Verification items for the finished model (mm, model axes). Round coordinates to 2 decimals unless told otherwise and drop trailing zeros. Write each loop counter-clockwise with the first axis right and the second up, starting at its lowest first coordinate (ties: lowest second). Pieces come first, ordered by that corner, then holes. Notation, with made-up numbers: (-37.75, -39.75) - (19.25, -39.75) arc R20 cw to (19.25, -12.75) - close; hole circle Ø1 at (27, 40.25). An arc over 180 degrees is marked (long way). Answer as a JSON object with one key per item and string values.
Autodesk Inventor part; units mm, degrees
ref_plane "YZ Plane" through (0, 0, 0) normal (1, 0, 0) x (0, 1, 0)
ref_plane "XZ Plane" through (0, 0, 0) normal (0, 1, 0) x (-1, 0, 0)
ref_plane "XY Plane" through (0, 0, 0) normal (0, 0, 1) x (1, 0, 0)
sketch "Sketch1" plane through (0, 0, 0) normal (0, 0, 1) x (1, 0, 0)
  line L0 (700, -200) -> (180, -200)
  line L1 (180, -200) -> (-160, -200)
  line L2 (-160, -200) -> (-160, 200)
  line L3 (180, -200) -> (180, 200)
  line L4 (700, -200) -> (1018.8395, -200)
  line L5 (1018.8395, -200) -> (1018.8395, 200)
  line L6 (1018.8395, 200) -> (700, 200)
  line L7 (180, 200) -> (700, 200)
  line L8 (-160, 200) -> (180, 200)
  line L9 (740, 160) -> (740, 200)
  line L10 (740, 160) -> (740, -160)
  line L11 (740, -200) -> (740, -160)
  line L12 (700, 160) -> (700, -160)
  line L13 (700, -160) -> (700, -200)
  line L14 (700, 200) -> (700, 160)
  line L15 (140, 160) -> (140, 200)
  line L16 (140, -200) -> (140, -160)
  line L17 (140, 160) -> (140, -160)
  line L18 (700, -160) -> (180, -160)
  line L19 (180, 160) -> (700, 160)
  line L20 (180, -200) -> (340, -200)
  line L21 (340, -200) -> (340, 0)
  line L22 (340, 0) -> (180, 0)
  line L23 (180, 0) -> (180, -200)
  point P0 (0, 0)
  point P1 (260, 0)
  point P2 (140, 0)
  dimension "d0" = 160
extrude "Extrusion1" add sketch "Sketch1" along normal blind 160 contours L0 L3 L18 L21 | L18 L3 L22 L21
ref_plane "Work Plane1" through (260, -200, 0) normal (1, 0, 0) x (0, 0, -1)
sketch "Sketch2" plane through (260, -200, 0) normal (1, 0, 0) x (0, 0, -1)
  line L0 (0, 200) -> (0, 0)
  line L1 (0, 0) -> (-160, 0)
  line L2 (-160, 200) -> (-160, 0)
  line L3 (0, 200) -> (-160, 200)
  line L4 (0, 0) -> (-160, 0)
  line L5 (-80, 0) -> (-80, 200)
  line L6 (0, 200) -> (-160, 200)
  line L7 (-74, 200) -> (-74, 220)
  line L8 (-74, 220) -> (-50, 220)
  line L9 (-50, 220) -> (-50, 228)
  line L10 (-50, 228) -> (-80, 228)
  line L11 (-80, 228) -> (-80, 200)
  line L12 (-80, 200) -> (-80, 294.9893)
  dimension "d6" = 8
  dimension "d7" = 12
  dimension "d8" = 20
  dimension "d9" = 30
  dimension "d10" = 94.9893
revolve "Revolution1" add sketch "Sketch2" angle 360 about axis through (260, 0, 80) along (0, 1, 0) contours L3 L11 L10 L9 L8 L7
properties part number "aandrijfMotor"
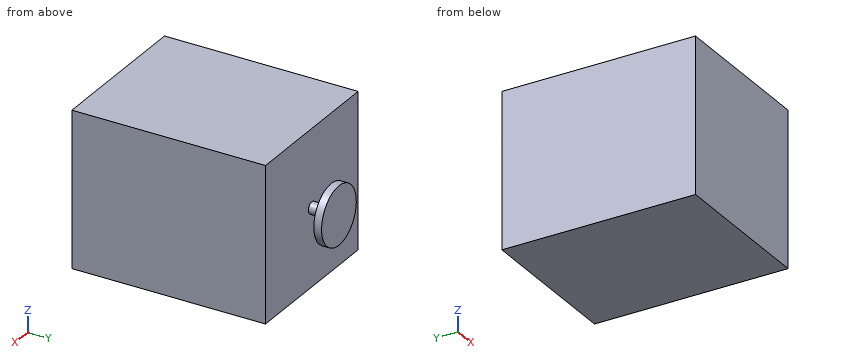
1. Material ranges on probe 1 along Y at (x, z) = (270, 106); probe 2 along Y at (x, z) = (219.5, 80); probe 3 along X at (y, z) = (15.5, 79), recorded low to high. Write a range as from..to.
Completed:
{"probe 1": "y = -200..0, 20..28", "probe 2": "y = -200..0", "probe 3": "x = 254.08..265.92"}
2. Cross-section at B-B (z = 59). Record the boundary of the cut face in (x, y).
Completed:
{"outline": "(180, -200) - (340, -200) - (340, 0) - (180, 0) - close; (238.58, 20) - (281.42, 20) - (281.42, 28) - (238.58, 28) - close"}
3. Cross-section at C-C (z = 80). Record the boundary of the cut face in (x, y), plus the area to 3 significant figures.
Completed:
{"outline": "(180, -200) - (340, -200) - (340, 0) - (266, 0) - (266, 20) - (290, 20) - (290, 28) - (230, 28) - (230, 20) - (254, 20) - (254, 0) - (180, 0) - close", "area": "32,700 mm^2"}
4. Cross-section at D-D (x = 203.5). Record the boundary of the cut face in (y, z), plus the area to 3 significant figures.
Completed:
{"outline": "(-200, 0) - (0, 0) - (0, 160) - (-200, 160) - close", "area": "32,000 mm^2"}
5. Cross-section at A-A (x = 250). Record the boundary of the cut face in (y, z), plus the area to 3 significant figures.
Completed:
{"outline": "(-200, 0) - (0, 0) - (0, 160) - (-200, 160) - close; (20, 51.72) - (28, 51.72) - (28, 108.28) - (20, 108.28) - close", "area": "32,500 mm^2"}
6. Go/stop test with a flat-tipped pin: pin 1 (4 mm diameter, centred on x = 261.5, y = -126.5, fed in from -Z). Record where the tip stops, or that it passes through.
Completed:
{"pin 1": "stops at z = 0"}
